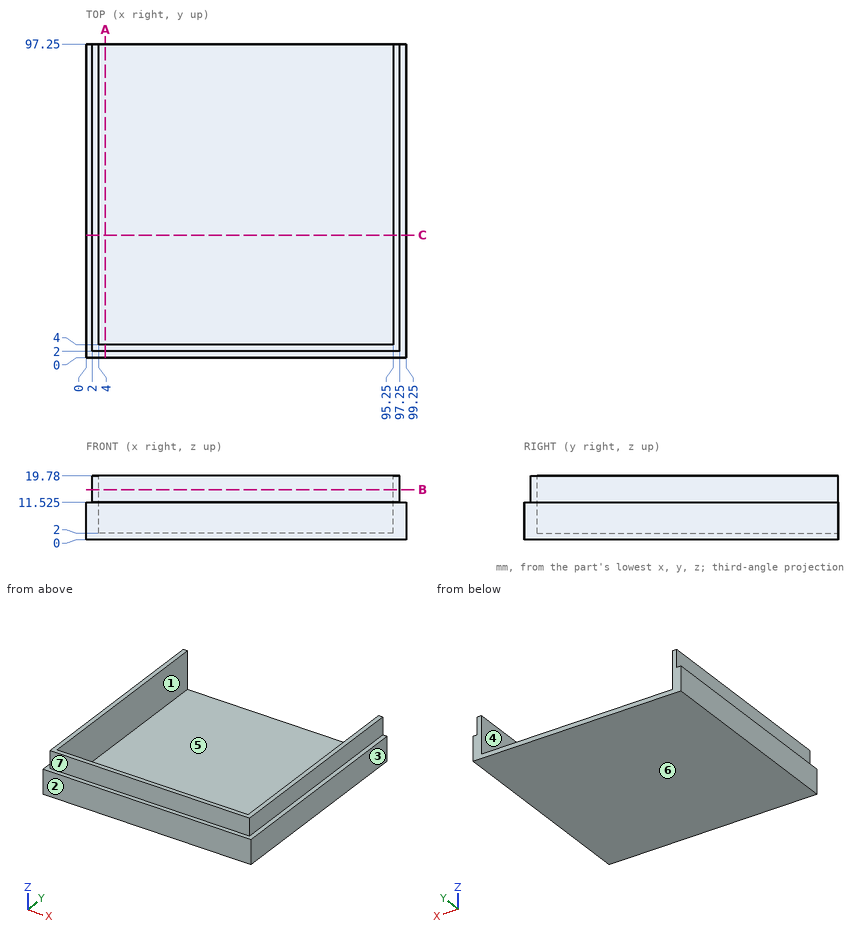
Check sheet for the drawn part. Datum: minimum x, y, z corner. Units: mm. A direction names the side the tool comes from. Give positions to 0.01 mm unless a question says otherwise; leave off trailing zeros. Order: outer loops, then holes, each group sorted by start corner. A loop starts at its lowest first (then second) coordinate and runs counter-clockwise, first axis right, second up. Notation, with made-up numbers: (70, 58) -> (125, 58) arc R29 cw to (125, 93) -> close; hole circle Ø1 at (27.25, -5). An arc over 180 degrees is marked (long way). Return JSON: item names as keys, results as strings.
1. Mould release check, pull along X, two halves, no side actions. Record for the marked faces 1, 2, 3 and 4: +X half, -X half, draft (parallel to the pull), parting line (faces both ways), or undercut.
From the geometry:
{"face 1": "undercut", "face 2": "draft", "face 3": "+X half", "face 4": "undercut"}
2. Set-up check for the marked faces 5, 6 and 7: record each of +Z, -Z, +X, -X, +Y, -Y from which the full face is reachable in a straight line by a thin tool's end or side.
From the geometry:
{"face 5": "+Z, +Y", "face 6": "-Z, +X, -X, +Y, -Y", "face 7": "+Z, +X, -X, -Y"}
3. Cross-section at C-C, the plane y = 38. Record the cut outline in (x, z) (3 decimals).
From the geometry:
{"outline": "(0, 0) -> (99.25, 0) -> (99.25, 11.525) -> (97.25, 11.525) -> (97.25, 19.78) -> (95.25, 19.78) -> (95.25, 2) -> (4, 2) -> (4, 19.78) -> (2, 19.78) -> (2, 11.525) -> (0, 11.525) -> close"}
4. Cross-section at A-A, the plane x = 6. Record the cut outline in (y, z) (3 decimals), plus the area to 3 significant figures.
From the geometry:
{"outline": "(0, 0) -> (97.25, 0) -> (97.25, 2) -> (4, 2) -> (4, 19.78) -> (2, 19.78) -> (2, 11.525) -> (0, 11.525) -> close", "area": "249 mm^2"}
5. Material ranges on probe 1 along X at (y, z) = (58.5, 18); probe 2 along X at (y, z) = (85, 6.5); probe 3 along Y at (x, z) = (49, 14), recorded low to high. Write a range as [from, to].
From the geometry:
{"probe 1": "[2, 4], [95.25, 97.25]", "probe 2": "[0, 4], [95.25, 99.25]", "probe 3": "[2, 4]"}
6. Cross-section at B-B, the plane z = 15.5. Record the cut outline in (x, y).
From the geometry:
{"outline": "(2, 2) -> (97.25, 2) -> (97.25, 97.25) -> (95.25, 97.25) -> (95.25, 4) -> (4, 4) -> (4, 97.25) -> (2, 97.25) -> close"}
7. Go/stop test with flat-tipped pins: P1, Ø6.5, axis at y = 52.5, z = 17, coming from the +X side; P2, Ø9, axis at x = 48.5, z = 12, coming from the +Y side; P3, Ø5, axis at x = 42.5, y = 65, coming from the +Z side. Record where each tip stops, or that it passes through.
From the geometry:
{"P1": "x = 97.25", "P2": "y = 4", "P3": "z = 2"}
